```python
from build123d import *

# Parameters (mm, degrees)
BOSS_EXTRUDE1_DEPTH      = 3
BOSS_EXTRUDE2_DEPTH      = 6
BOSS_EXTRUDE2_DEPTH_BACK = 5.2
CHAMFER1_SIZE            = 0.1


with BuildPart() as part:
    # Sketch2 → Boss-Extrude1 (new body)
    with BuildSketch(Plane(origin=(0, 0, 0), x_dir=(1, 0, 0), z_dir=(0, 1, 0))):
        Polygon((-1.25, -1.05), (-1.05, -1.25), (1.05, -1.25), (1.25, -1.05), (1.45, -1.25), (3.55, -1.25), (3.75, -1.05), (3.75, 1.05), (3.55, 1.25), (1.45, 1.25), (1.25, 1.05), (1.05, 1.25), (-1.05, 1.25), (-1.25, 1.05), (-1.45, 1.25), (-3.55, 1.25), (-3.75, 1.05), (-3.75, -1.05), (-3.55, -1.25), (-1.45, -1.25), align=None)
    extrude(amount=BOSS_EXTRUDE1_DEPTH)

    # Sketch3 → Boss-Extrude2 (add, two sides: drawn at the far end of the back side and taken through both)
    with BuildSketch(Plane(origin=(0, 3, 0), x_dir=(1, 0, 0), z_dir=(0, 1, 0)).offset(-BOSS_EXTRUDE2_DEPTH_BACK)):
        Polygon((0.3, 0.31), (-0.3, 0.31), (-0.31, 0.3), (-0.31, -0.3), (-0.3, -0.31), (0.3, -0.31), (0.31, -0.3), (0.31, 0.3), align=None)
        Polygon((-2.2, -0.31), (-2.19, -0.3), (-2.19, 0.3), (-2.2, 0.31), (-2.8, 0.31), (-2.81, 0.3), (-2.81, -0.3), (-2.8, -0.31), align=None)
        Polygon((2.8, -0.31), (2.81, -0.3), (2.81, 0.3), (2.8, 0.31), (2.2, 0.31), (2.19, 0.3), (2.19, -0.3), (2.2, -0.31), align=None)
    extrude(amount=BOSS_EXTRUDE2_DEPTH + BOSS_EXTRUDE2_DEPTH_BACK)

    # Chamfer1
    # the kernel refuses this chamfer: 0.1 mm, written as the material it takes off along each edge
    with BuildSketch(Plane(origin=(-2.81, 9, -0.557168299), x_dir=(-0.027495876610587656, -0.9996219169112966, 0), z_dir=(0, 0, 1)), Plane(origin=(-1.942831701, 9, -0.31), x_dir=(0, -0.9996219169112968, -0.02749587661058658), z_dir=(-1, 0, 0)), Plane(origin=(-2.19, 9, 0.557168299), x_dir=(0.027495876610587656, -0.9996219169112966, 0), z_dir=(0, 0, -1)), Plane(origin=(-3.057168299, 9, 0.31), x_dir=(0, -0.9996219169112968, 0.02749587661058658), z_dir=(1, 0, 0)), Plane(origin=(2.19, 9, -0.557168299), x_dir=(-0.027495876610587656, -0.9996219169112966, 0), z_dir=(0, 0, 1)), Plane(origin=(3.057168299, 9, -0.31), x_dir=(0, -0.9996219169112968, -0.02749587661058658), z_dir=(-1, 0, 0)), Plane(origin=(2.81, 9, 0.557168299), x_dir=(0.027495876610587656, -0.9996219169112966, 0), z_dir=(0, 0, -1)), Plane(origin=(1.942831701, 9, 0.31), x_dir=(0, -0.9996219169112968, 0.02749587661058658), z_dir=(1, 0, 0)), Plane(origin=(0.557168299, 9, -0.31), x_dir=(0, -0.9996219169112968, -0.02749587661058658), z_dir=(-1, 0, 0)), Plane(origin=(0.31, 9, 0.557168299), x_dir=(0.027495876610586577, -0.9996219169112966, 0), z_dir=(0, 0, -1)), Plane(origin=(-0.557168299, 9, 0.31), x_dir=(0, -0.9996219169112968, 0.02749587661058658), z_dir=(1, 0, 0)), Plane(origin=(-0.31, 9, -0.557168299), x_dir=(-0.027495876610586577, -0.9996219169112966, 0), z_dir=(0, 0, 1))) as chamfer1_piece_1:
        Polygon((CHAMFER1_SIZE * 0.999621916911, CHAMFER1_SIZE * 0.0274958766106), (-CHAMFER1_SIZE * 0.0274958766106, CHAMFER1_SIZE * 0.999621916911), (0, 0), align=None)
    extrude(amount=1.114336598, mode=Mode.SUBTRACT)
    with BuildSketch(Plane(origin=(2.81, -2.2, 0.557168299), x_dir=(0.02749587661058718, 0.9996219169112966, 0), z_dir=(0, 0, -1)), Plane(origin=(3.057168299, -2.2, -0.31), x_dir=(0, 0.9996219169112968, -0.027495876610586105), z_dir=(-1, 0, 0)), Plane(origin=(2.19, -2.2, -0.557168299), x_dir=(-0.02749587661058718, 0.9996219169112966, 0), z_dir=(0, 0, 1)), Plane(origin=(1.942831701, -2.2, 0.31), x_dir=(0, 0.9996219169112968, 0.027495876610586105), z_dir=(1, 0, 0)), Plane(origin=(-0.31, -2.2, -0.557168299), x_dir=(-0.027495876610586105, 0.9996219169112968, 0), z_dir=(0, 0, 1)), Plane(origin=(-0.557168299, -2.2, 0.31), x_dir=(0, 0.9996219169112968, 0.027495876610586105), z_dir=(1, 0, 0)), Plane(origin=(0.31, -2.2, 0.557168299), x_dir=(0.027495876610586105, 0.9996219169112968, 0), z_dir=(0, 0, -1)), Plane(origin=(0.557168299, -2.2, -0.31), x_dir=(0, 0.9996219169112968, -0.027495876610586105), z_dir=(-1, 0, 0)), Plane(origin=(-2.19, -2.2, 0.557168299), x_dir=(0.02749587661058718, 0.9996219169112966, 0), z_dir=(0, 0, -1)), Plane(origin=(-1.942831701, -2.2, -0.31), x_dir=(0, 0.9996219169112968, -0.027495876610586105), z_dir=(-1, 0, 0)), Plane(origin=(-2.81, -2.2, -0.557168299), x_dir=(-0.02749587661058718, 0.9996219169112966, 0), z_dir=(0, 0, 1)), Plane(origin=(-3.057168299, -2.2, 0.31), x_dir=(0, 0.9996219169112968, 0.027495876610586105), z_dir=(1, 0, 0))) as chamfer1_piece_2:
        Polygon((CHAMFER1_SIZE * 0.999621916911, -CHAMFER1_SIZE * 0.0274958766106), (-CHAMFER1_SIZE * 0.0274958766106, -CHAMFER1_SIZE * 0.999621916911), (0, 0), align=None)
    extrude(amount=1.114336598, mode=Mode.SUBTRACT)


solid = part.part
```
Geometry: final body of the model. Coordinates: model frame, mm. A direction names the side the tool comes from. Round coordinates to 2 decimals unless told otherwise and drop trailing zeros. Write each loop counter-clockwise with the first axis right and the second up, starting at its lowest first coordinate (ties: lowest second). Pieces come first, ordered by that corner, then holes. Notation, with made-up numbers: (24, 82) -> (54, 82) arc R32 ccw to (54, 114) -> close; hole circle Ø9 at (-30, 87.5). An arc over 180 degrees is marked (long way). Return JSON: item names as keys, results as strings.
Q1. Section B-B on x = 2.5. Return the cut outline in (y, z).
From the geometry:
{"outline": "(-2.2, -0.21) -> (-2.1, -0.31) -> (0, -0.31) -> (0, -1.25) -> (3, -1.25) -> (3, -0.31) -> (8.9, -0.31) -> (9, -0.21) -> (9, 0.21) -> (8.9, 0.31) -> (3, 0.31) -> (3, 1.25) -> (0, 1.25) -> (0, 0.31) -> (-2.1, 0.31) -> (-2.2, 0.21) -> close"}
Q2. Section A-A on y = 5.25. Give the number of separate pieces and of enclosed holes in the cut face, and give its area (3 significant figures).
From the geometry:
{"separate pieces": "3", "enclosed holes": "0", "area": "1.15 mm2"}
Q3. Section C-C on z = -0.7. Return the cut outline in (x, y).
From the geometry:
{"outline": "(-3.75, 0) -> (3.75, 0) -> (3.75, 3) -> (-3.75, 3) -> close"}
Q4. Mould query, pull axis X, two halves, no side actions, for faces 3 (the flat face through (0, 3, -1)), 4 (the flat face through (3.75, 1, 0)), 5 (the flat face through (2, 1, 1.25)). Classes: +X half, -X half, draft (parallel to the pull), parting line (faces both ways), or undercut.
From the geometry:
{"face 3": "undercut", "face 4": "+X half", "face 5": "draft"}
Q5. First-contact query: pin 1 Ø0.5 at (x, y) = (0, -0.5) entering from +Z; pin 2 Ø1 at (x, y) = (-1, 7) entering from -Z; pin 3 Ø0.7 at (x, y) = (-2.5, -1.5) entering from -Z; pin 4 Ø0.5 at (y, z) = (6.5, 0) entering from -X. Flat tips, straight axial feed; report the tip coordinate or a pass-through.
From the geometry:
{"pin 1": "z = 0.31", "pin 2": "through", "pin 3": "z = -0.31", "pin 4": "x = -2.81"}
Q6. Set-up query: faces 1 (the flat face through (0, 0, -1)), 2 (the flat face through (3, 1, -1.25)). Return all of +Z, -Z, +X, -X, +Y, -Y with unobstructed straight access to the full face (end or side cutting, diameter ignored); none if empty.
From the geometry:
{"face 1": "-Y", "face 2": "-Z, +X, -X, +Y, -Y"}
Q7. Section D-D on x = 0.75. Return the cut outline in (y, z), and give its area (3 significant figures).
From the geometry:
{"outline": "(0, -1.25) -> (3, -1.25) -> (3, 1.25) -> (0, 1.25) -> close", "area": "7.50 mm2"}
Q8. Ray query, line 1 (X direction, y = 5, z = -0.1); line 2 (Y direction, x = -0.25, z = -0.85); line 3 (Z direction, x = 2.75, y = -1.25). Return the intervals inside material, ascending.
From the geometry:
{"line 1": "-2.81 to -2.19, -0.31 to 0.31, 2.19 to 2.81", "line 2": "0 to 3", "line 3": "-0.31 to 0.31"}
